Geometry check sheet. Reference: the model listing, model coordinates, mm. Round coordinates to 2 decimals unless told otherwise and drop trailing zeros. Write each loop counter-clockwise with the first axis right and the second up, starting at its lowest first coordinate (ties: lowest second). Pieces come first, ordered by that corner, then holes. Notation, with made-up numbers: M -30.5,53 L -4.5,53 A10 ccw -4.5,72 Z; hole C 63,84.5 d9. An arc over 180 degrees is marked long. Use a Markdown table: item, result.
Autodesk Inventor part; units mm, degrees
ref_plane "Start Plane" through (0, 0, 15) normal (0, 0, 1) x (1, 0, 0)
ref_plane "End Plane" through (0, 0, 535.0007) normal (0, 0, 1) x (1, 0, 0)
ref_plane "Work Plane4" through (9, 1515, 15) normal (0, 0, -1) x (-1, 0, 0)
ref_plane "Start Plane" through (0, 0, 15) normal (0, 0, 1) x (1, 0, 0)
ref_plane "End Plane" through (0, 0, 535.0007) normal (0, 0, 1) x (1, 0, 0)
sketch "Sketch" plane through (0, 0, 0) normal (0, 0, 1) x (1, 0, 0)
  line L0 (-15, -9) -> (-15, 9)
  line L1 (-9, 15) -> (9, 15)
  line L2 (15, 9) -> (15, -9)
  line L3 (9, -15) -> (-9, -15)
  arc A0 (-15, -9) -> (-9, -15) centre (-9, -9) ccw
  arc A1 (-9, 15) -> (-15, 9) centre (-9, 9) ccw
  arc A2 (15, 9) -> (9, 15) centre (9, 9) ccw
  arc A3 (9, -15) -> (15, -9) centre (9, -9) ccw
  arc A4 (-9, 12) -> (-12, 9) centre (-9, 9) ccw
  line L4 (-9, 12) -> (9, 12)
  arc A5 (12, 9) -> (9, 12) centre (9, 9) ccw
  line L5 (12, 9) -> (12, -9)
  arc A6 (9, -12) -> (12, -9) centre (9, -9) ccw
  line L6 (9, -12) -> (-9, -12)
  arc A7 (-12, -9) -> (-9, -12) centre (-9, -9) ccw
  line L7 (-12, -9) -> (-12, 9)
  line L8 (0, 22.7397) -> (0, -22.7397) construction
  line L9 (-22.7397, 0) -> (22.7397, 0) construction
  dimension "d7" = 6
  dimension "d10" = 30
  dimension "d11" = 30
  dimension "d12" = 3
  dimension "d15" = 15
  dimension "d16" = 15
extrude "Body" add sketch "Sketch" along normal up to surface (520.0007 mm away) from surface at 15
sketch "Sketch3" plane through (0, 0, 0) normal (0, 0, 1) x (1, 0, 0)
  line L0 (0, 0) -> (10, 0)
ref_plane "Work Plane3" through (0, 0, 0) normal (0, -1, 0) x (1, 0, 0)
ref_plane "Work Plane4" through (9, 1515, 15) normal (0, 0, -1) x (-1, 0, 0)
split "Split1" plane through (9, 1515, 15) removes the side toward (0, 0, -1)
ref_plane "Work Plane6" through (9.0011, 375, 535.0007) normal (0, 0, 1) x (1, 0, 0)
split "Split3" plane through (9.0011, 375, 535.0007) removes the side toward (0, 0, 1)
sketch "Sketch4" plane through (0, 0, 0) normal (0, -1, 0) x (1, 0, 0)
  line L0 (-2, 15) -> (12, 15)
  line L1 (-2, 535.0007) -> (12, 535.0007)
  dimension "d18" = 520.0007
equation "\"d7\" = G_IR"
equation "\"d10\" = G_H"
equation "\"d11\" = G_W"
equation "\"d12\" = G_T"
equation "\"d15\" = 0.5 * d10"
equation "\"d16\" = 0.5 * d11"
equation "\"d3\" = G_L"
equation "\"G_W\" = 30"
equation "\"G_H\" = 30"
equation "\"G_T\" = 3"
equation "\"G_IR\" = 6"
equation "\"G_L\" = d18"
equation "\"G_OFFSET_START\" = -15"
equation "\"G_OFFSET_END\" = -14.99934"
equation "\"d13\" = -G_OFFSET_START"
equation "\"d14\" = G_OFFSET_END + B_L"
properties part number "DIN EN 10219-2 - 30 x 30 x 3  - 520" material "Steel, Mild"
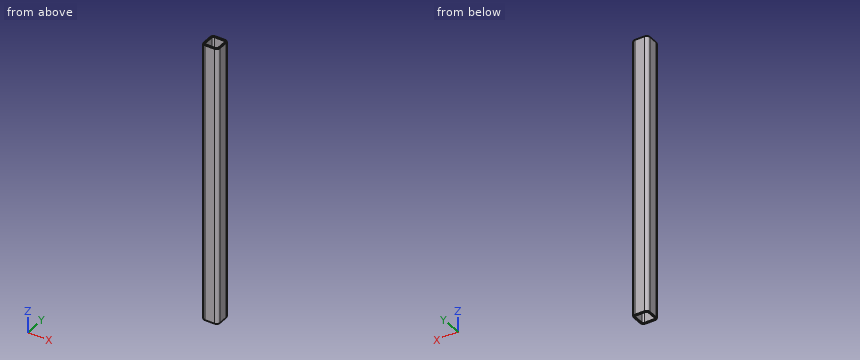
Item 1: Go/stop test with flat-tipped pins: pin 1 (4 mm diameter, centred on x = 10.5, y = -3.5, fed in from +Z); pin 2 (10 mm diameter, centred on x = 5.5, y = -6, fed in from +Z). Record where each tip stops, or that it passes through.
Outcome:
| item | result |
|---|---|
| pin 1 | stops at z = 535 |
| pin 2 | passes through |
Item 2: Material ranges on line 1 along Y through (x, z) = (-3.75, 345.5); line 2 along X through (y, z) = (-9.75, 195.5), recorded low to high. Write a range as from..to.
Outcome:
| item | result |
|---|---|
| line 1 | y = -15..-12, 12..15 |
| line 2 | x = -14.95..-11.9, 11.9..14.95 |
Item 3: Cross-section at A-A, the plane y = -2. Record the cut outline in (x, z), and give its area (3 significant figures).
Outcome:
| item | result |
|---|---|
| outline | M -15,15 L -12,15 L -12,535 L -15,535 Z; M 12,15 L 15,15 L 15,535 L 12,535 Z |
| area | 3,120 mm2 |
Item 4: Cross-section at B-B, the plane z = 47.5. Record the cut outline in (x, y).
Outcome:
| item | result |
|---|---|
| outline | M -15,-9 A6 ccw -9,-15 L 9,-15 A6 ccw 15,-9 L 15,9 A6 ccw 9,15 L -9,15 A6 ccw -15,9 Z; hole M -12,-9 A3 ccw -9,-12 L 9,-12 A3 ccw 12,-9 L 12,9 A3 ccw 9,12 L -9,12 A3 ccw -12,9 Z |
